from build123d import *

# Parameters (mm, degrees)
F0_W     = 340
F0_H     = 40
F1_DEPTH = 6
F2_W     = 180
F2_H     = 3
F3_DEPTH = 6
F5_D     = 6
F6_W     = 180
F6_H     = 10
F7_DEPTH = 6
F8_W     = 180
F8_H     = 1.6
F9_DEPTH = 4


with BuildPart() as f1:
    # F0 (on Right) → F1 (new body, symmetric)
    with BuildSketch(Plane.YZ):
        with Locations((170, 20)):
            Rectangle(F0_W, F0_H)
    extrude(amount=F1_DEPTH, both=True)

    # F2 (on face) → F3 (cut)
    with BuildSketch(Plane.YZ.offset(6)):
        with Locations((250, 33.5)):
            Rectangle(F2_W, F2_H)
    extrude(amount=-F3_DEPTH, mode=Mode.SUBTRACT)

    # F5 (through all)
    with Locations(Plane.YZ.offset(6)):
        with Locations((116.477057, 20)):
            Hole(F5_D / 2)

    # F6 (on face) → F7 (cut)
    with BuildSketch(Plane.YZ.offset(6)):
        with Locations((250, 21)):
            Rectangle(F6_W, F6_H)
    extrude(amount=-F7_DEPTH, mode=Mode.SUBTRACT)

    # F8 (on face) → F9 (cut)
    with BuildSketch(Plane.YZ.offset(6)):
        with Locations((250, 6.862387)):
            Rectangle(F8_W, F8_H)
    extrude(amount=-F9_DEPTH, mode=Mode.SUBTRACT)


solid = f1.part
The model under review builds one solid part; all positions refer to its coordinate system, in mm. A direction names the side the tool comes from. Round coordinates to 2 decimals unless told otherwise and drop trailing zeros. Write each loop counter-clockwise with the first axis right and the second up, starting at its lowest first coordinate (ties: lowest second). Pieces come first, ordered by that corner, then holes. Notation, with made-up numbers: (-11, 20.25) - (4, 20.25) arc R32 ccw to (4, 55.25) - close; hole circle Ø8 at (-18.75, 82). An arc over 180 degrees is marked (long way). One line per item, written item: value. Start each with the question number.
1. Consider section C-C on y = 227.5. Write out the cut boundary in (x, z).
2. To check wall thickness, follow L1, parallel to Z at x = 5.75, y = 311.5; L2, parallel to X at y = 307.5, z = 25.5; L3, parallel to X at y = 290, z = 6.5. State the ranges of each line that lie inside material, in increasing order. Write a range as from..to.
3. The part is to be moulded in two halves that separate along Y. For faces 1 (the face through (-0.084, 113.616, 20.901)), 2 (the face through (3, 249, 26)), 3 (the face through (0, 0, 20)), say which applies: released by +Y, released by -Y, zero draft, split by the parting line, or undercut.
4. Consider section A-A on z = 20. Write out the cut boundary in (x, y).
5. Consider section B-B on x = 4. Write out the cut boundary in (y, z), and give its area (3 significant figures).
6. Clearance check with flat-ended pins moving along their axes: P1, Ø1.8, axis at x = 4, z = 19, coming from the +Y side; P2, Ø2.5, axis at y = 252, z = 33.5, coming from the +X side. State where each tip first meets the part, or that it passes through.
7. Machinability: for faces 4 (the face through (3, 249, 32)), 5 (the face through (-6, 168, 20)), which of the approach directions +Z, -Z, +X, -X, +Y, -Y give a long, thin tool a straight path to every point of the face, cutting with its end or side? Answer none if there is none.
Checks:
1. outline: (-6, 0) - (6, 0) - (6, 6.06) - (2, 6.06) - (2, 7.66) - (6, 7.66) - (6, 16) - (0, 16) - (0, 26) - (6, 26) - (6, 32) - (0, 32) - (0, 35) - (6, 35) - (6, 40) - (-6, 40) - close
2. L1: z = 0..6.06, 7.66..16, 26..32, 35..40
2. L2: x = -6..0
2. L3: x = -6..2
3. face 1: undercut
3. face 2: zero draft
3. face 3: released by -Y
4. outline: (-6, 0) - (6, 0) - (6, 113.48) - (-6, 113.48) - close; (-6, 119.48) - (6, 119.48) - (6, 160) - (0, 160) - (0, 340) - (-6, 340) - close
5. outline: (0, 0) - (340, 0) - (340, 6.06) - (160, 6.06) - (160, 7.66) - (340, 7.66) - (340, 16) - (160, 16) - (160, 26) - (340, 26) - (340, 32) - (160, 32) - (160, 35) - (340, 35) - (340, 40) - (0, 40) - close; hole circle Ø6 at (116.48, 20)
5. area: 10,900 mm^2
6. P1: stops at y = 160
6. P2: stops at x = 0
7. face 4: +X, +Y
7. face 5: +Z, -Z, -X, +Y, -Y
